Verification items for the finished model (mm, model axes). Face numbers are marked on the shaded views. A direction names the side the tool comes from. Coordinates: 2 decimals unless noted, no trailing zeros. Order: outer loops, then holes, each group sorted by start corner. A loop starts at its lowest first (then second) coordinate and runs counter-clockwise, first axis right, second up. Notation, with made-up numbers: (18.25, 28.25) -> (45.25, 28.25) arc R32 ccw to (45.25, 64.25) -> close; hole circle Ø9 at (45.5, 27.5). An arc over 180 degrees is marked (long way). Write each question's results on one line, items separated by ' | '. Start each with the question number.
(1) Set-up check for the marked faces 1 and 2: record each of +Z, -Z, +X, -X, +Y, -Y from which the full face is reachable in a straight line by a thin tool's end or side.
(2) Thickness scan on probe 1 along Z at (x, y) = (9, 1.15); probe 2 along X at (y, z) = (12, -2.5). Record the ranges inside material, lowest first. Write a range as [from, to].
(3) Cross-section at B-B on z = -15. Enter the section's corners in (x, y), and give its area (4 significant figures).
(4) Cross-section at D-D on x = 2. Enter the section's corners in (y, z).
(5) Cross-section at A-A on y = 10. Enter the section's corners in (x, z), and give its area (3 significant figures).
(6) Cross-section at C-C on x = 8. Enter the section's corners in (y, z).
(7) Go/stop test with flat-tipped pins: pin 1 (3 mm diameter, centred on x = 5, z = -8, fed in from +Y); pin 2 (5 mm diameter, centred on y = 12, z = -2.5, fed in from +X). Record where each tip stops, or that it passes through.
```python
from build123d import *

# Parameters (mm, degrees)
EXTRUDE_THIN1_DEPTH = 20
SKETCH2_R           = 2.5
CUT_EXTRUDE1_DEPTH  = 21
SKETCH3_R           = 2.5
CUT_EXTRUDE2_DEPTH  = 2.5


with BuildPart() as part:
    # Sketch1 → Extrude-Thin1 (new body)
    with BuildSketch(Plane.XY):
        Polygon((0, 20), (0, 0), (20, 0), (20, 1.5), (1.5, 1.5), (1.5, 20), align=None)
    extrude(amount=EXTRUDE_THIN1_DEPTH)

    # Sketch2 → Cut-Extrude1 (cut, through all)
    with BuildSketch(Plane(origin=(0, 0, 0), x_dir=(-1, 0, 0), z_dir=(0, -1, 0))):
        with Locations((-9, -15)):
            Circle(SKETCH2_R)
    extrude(amount=-CUT_EXTRUDE1_DEPTH, mode=Mode.SUBTRACT)

    # Sketch3 → Cut-Extrude2 (cut, through all)
    with BuildSketch(Plane(origin=(1.5, 0, 0), x_dir=(0, 0, -1), z_dir=(1, 0, 0))):
        with Locations((-7, 10)):
            Circle(SKETCH3_R)
    extrude(amount=-CUT_EXTRUDE2_DEPTH, mode=Mode.SUBTRACT)


with BuildPart() as body_2:
    # Mirror1: mirrored copy
    add(part.part.mirror(Plane.XY))


solid = body_2.part
```
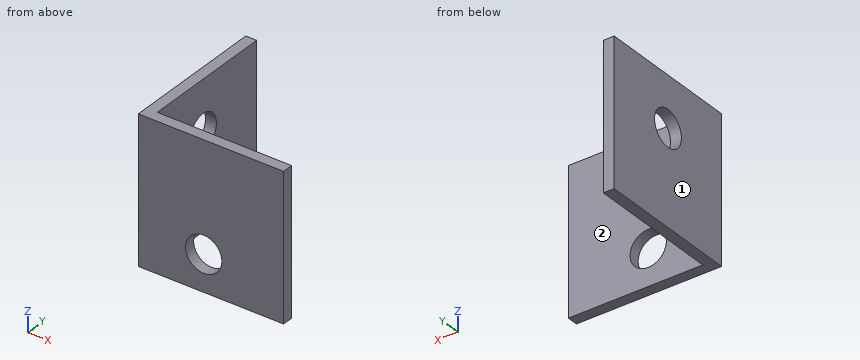
Results are:
1) face 1: +Z, -Z, -X, +Y, -Y | face 2: +Z, -Z, +X, +Y
2) probe 1: z = [-20, -17.5], [-12.5, 0] | probe 2: x = [0, 1.5]
3) outline: (0, 0) -> (6.5, 0) -> (6.5, 1.5) -> (1.5, 1.5) -> (1.5, 20) -> (0, 20) -> close; (11.5, 0) -> (20, 0) -> (20, 1.5) -> (11.5, 1.5) -> close | area: 50.25 mm2
4) outline: (0, -20) -> (1.5, -20) -> (1.5, 0) -> (0, 0) -> close
5) outline: (0, -20) -> (1.5, -20) -> (1.5, -9.5) -> (0, -9.5) -> close; (0, -4.5) -> (1.5, -4.5) -> (1.5, 0) -> (0, 0) -> close | area: 22.5 mm2
6) outline: (0, -20) -> (1.5, -20) -> (1.5, -17.29) -> (0, -17.29) -> close; (0, -12.71) -> (1.5, -12.71) -> (1.5, 0) -> (0, 0) -> close
7) pin 1: stops at y = 1.5 | pin 2: stops at x = 1.5
